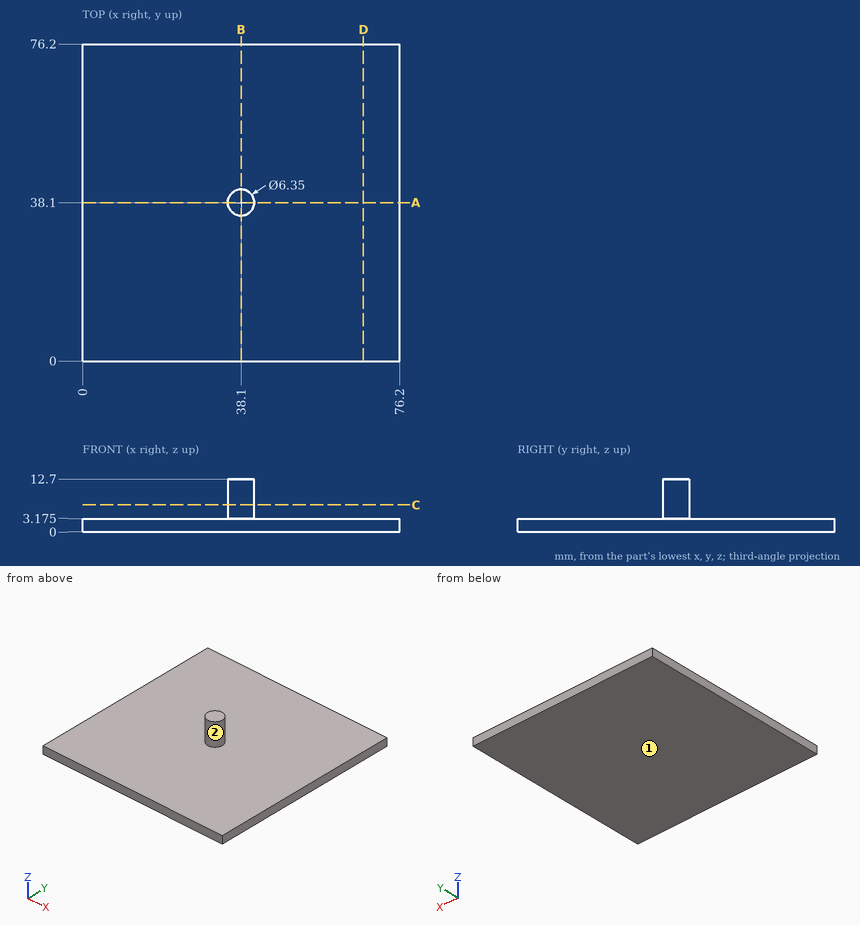
Input: dimensioned drawing with shaded views. Units: mm. Origin: part minimum x, y, z. A direction names the side the tool comes from. Round coordinates to 2 decimals unless told otherwise and drop trailing zeros. Loops run counter-clockwise (first coordinate to the right, second up) from the corner with the lowest first, then second, coordinate; pieces in that order, holes last. Notation, with made-up numbers: (22, -25.75) -> (69, -25.75) arc R22 ccw to (69, 3.25) -> close; hole circle Ø7 at (-17.5, -0.5). An arc over 180 degrees is marked (long way). Answer as a JSON object with one key per item and string values. Group by question number.
1) Section query C-C on z = 6.5. Output: boundary loops of the cut face in (x, y) (3 decimals).
2) Pin query (flat end, axial travel): pin 1 (1 mm diameter, centred on x = 12, y = 11, fed in from +Z) (3 decimals). Return the tip coordinate at first contact, or that it passes through.
3) Reachability of the marked faces 1 and 2 from +Z, -Z, +X, -X, +Y, -Y: full face, straight path, thin tool, end or side. Return the list, or none.
4) Section query A-A on y = 38.1. Output: boundary loops of the cut face in (x, z) (3 decimals), plus the area to 3 significant figures.
5) Ray query, L1, parallel to Z at x = 42, y = 21 (3 decimals). Return the intervals inside material, ascending.
6) Section query D-D on x = 67.5. Output: boundary loops of the cut face in (y, z) (3 decimals), plus the area to 3 significant figures.
Reply:
{
 "1": {"outline": "circle Ø6.35 at (38.1, 38.1)"},
 "2": {"pin 1": "stops at z = 3.175"},
 "3": {"face 1": "-Z, +X, -X, +Y, -Y", "face 2": "+Z"},
 "4": {"outline": "(0, 0) -> (76.2, 0) -> (76.2, 3.175) -> (41.275, 3.175) -> (41.275, 12.7) -> (34.925, 12.7) -> (34.925, 3.175) -> (0, 3.175) -> close", "area": "302 mm2"},
 "5": {"L1": "z = 0 to 3.175"},
 "6": {"outline": "(0, 0) -> (76.2, 0) -> (76.2, 3.175) -> (0, 3.175) -> close", "area": "242 mm2"}
}
